from build123d import *

# Parameters (mm, degrees)
F1_DEPTH = 2
F2_SIZE  = 1


with BuildPart() as f1:
    # F0 (on Top) → F1 (new body, symmetric)
    with BuildSketch(Plane.XY):
        with BuildLine():
            Line((-64.3336782856, 36.2610286334), (-64.3336782856, 34.8834841531))
            Line((-64.3336782856, 34.8834841531), (-57.4157565349, 34.8834841531))
            Line((-57.4157565349, 34.8834841531), (-57.4157565349, 36.4834841531))
            ThreePointArc((-57.4157565349, 36.4834841531), (-56.2994751301, 38.665413461), (-55.5534152324, 41))
            Line((-55.5534152324, 41), (-53.1534152324, 41))
            Line((-53.1534152324, 41), (-53.1534152324, 42.5))
            Line((-53.1534152324, 42.5), (-43.6123318144, 42.5))
            Line((-43.6123318144, 42.5), (-43.6123318144, 45))
            Line((-43.6123318144, 45), (-43.6123318144, 47.5))
            Line((-43.6123318144, 47.5), (-53.1534152324, 47.5))
            Line((-53.1534152324, 47.5), (-53.1534152324, 49))
            Line((-53.1534152324, 49), (-55.5534152324, 49))
            ThreePointArc((-55.5534152324, 49), (-56.2994751301, 51.334586539), (-57.4157565349, 53.5165158469))
            Line((-57.4157565349, 53.5165158469), (-57.4157565349, 55.1165158469))
            Line((-57.4157565349, 55.1165158469), (-64.3336782856, 55.1165158469))
            Line((-64.3336782856, 55.1165158469), (-64.3336782856, 53.7389713666))
            ThreePointArc((-64.3336782856, 53.7389713666), (-61.2693193587, 50.1809672734), (-60.1668349206, 45.6165158469))
            Line((-60.1668349206, 45.6165158469), (-60.1668349206, 44.3834841531))
            ThreePointArc((-60.1668349206, 44.3834841531), (-61.2693193587, 39.8190327266), (-64.3336782856, 36.2610286334))
        make_face()
    extrude(amount=F1_DEPTH, both=True)

    # F2
    f2_edges = [f1.edges().sort_by_distance(p)[0] for p in [
        (-54.353415, 49, -2),
        (-54.353415, 49, 2),
        (-54.353415, 41, 2),
        (-54.353415, 41, -2),
        (-48.382874, 47.5, -2),
        (-48.382874, 42.5, -2),
        (-48.382874, 47.5, 2),
        (-48.382874, 42.5, 2),
        (-61.269319, 50.180967, 2),
        (-61.269319, 39.819033, -2),
        (-61.269319, 39.819033, 2),
        (-60.166835, 45, -2),
        (-60.166835, 45, 2),
        (-61.269319, 50.180967, -2),
    ]]
    chamfer(f2_edges, length=F2_SIZE)


solid = f1.part
Part model, mm, in its own coordinate system. A direction names the side the tool comes from. Coordinates: 2 decimals unless noted, no trailing zeros. Loops run counter-clockwise (first coordinate to the right, second up) from the corner with the lowest first, then second, coordinate; pieces in that order, holes last. Notation, with made-up numbers: (62, -31) -> (117, -31) arc R8 cw to (117, -19) -> close; hole circle Ø7 at (78, 44.25). An arc over 180 degrees is marked (long way). Use a Markdown table: item, result. Add a question column.
Item 1: Band-saw the part on A-A on x = -54.25. Write the cut outline in (y, z), plus the area to 3 significant figures.
Item 2: Which spindle directions (+Z, -Z, +X, -X, +Y, -Y) get a long thin tool onto all of the face, cutting with end or side? Do faces 5 (the flat face through (-48.4, 43, 1.5)), 6 (the flat face through (-54.3, 48.5, -1.5)), 7 (the flat face through (-48.4, 43, -1.5)), 8 (the flat face through (-54, 41, 0)), 9 (the flat face through (-60.167, 45, 0)). Say none if no direction does.
Item 3: Flat gauge pins, fed straight in: P1, Ø0.6, axis at x = -54.5, z = -0.5, coming from the +Y side; P2, Ø1, axis at x = -46.5, z = 0.5, coming from the +Y side; P3, Ø2, axis at y = 43, z = 0, coming from the -X side. Where does each tip first touch, or does it go through?
Item 4: Probe probe 1 along Y at (x, z) = (-55.5, 0.6); probe 2 along Y at (x, z) = (-45, 0); probe 3 along Y at (x, z) = (-62, 0.8). List the from-to ranges inside material, lowest first.
Item 5: Pull direction Y, two halves, no side cores. Call faces 1 (the flat face through (-54, 49, 0)), 2 (the flat face through (-57.416, 54, 0)), 3 (the cylindrical face through (-61.24, 39.88, 0.01)), 4 (the conical face through (-61.1, 39.5, 1.3)): +Y half, -Y half, draft (parallel to the pull), parting line (faces both ways), or undercut.
Item 6: Band-saw the part on C-C on z = 1.75. Write the cut outline in (x, y), plus the area to 3 significant figures.
Item 7: Band-saw the part on B-B on z = -0.05. Write the cut outline in (x, y).
Geometry says:
| question | item | result |
|---|---|---|
| 1 | outline | (41, -1) -> (42, -2) -> (48, -2) -> (49, -1) -> (49, 1) -> (48, 2) -> (42, 2) -> (41, 1) -> close |
| 1 | area | 30.0 mm² |
| 2 | face 5 | +Z, +X, -Y |
| 2 | face 6 | -Z, +X, +Y |
| 2 | face 7 | -Z, +X, -Y |
| 2 | face 8 | +Z, -Z, +X, -Y |
| 2 | face 9 | +Z, -Z, -X |
| 3 | P1 | y = 49 |
| 3 | P2 | y = 47.5 |
| 3 | P3 | x = -60.46 |
| 4 | probe 1 | 41 to 49 |
| 4 | probe 2 | 42.5 to 47.5 |
| 4 | probe 3 | 34.88 to 38.61, 51.39 to 55.12 |
| 5 | face 1 | +Y half |
| 5 | face 2 | draft |
| 5 | face 3 | undercut |
| 5 | face 4 | undercut |
| 6 | outline | (-64.33, 34.88) -> (-57.42, 34.88) -> (-57.42, 36.48) arc R15 ccw to (-55.4, 41.75) -> (-53.15, 41.75) -> (-53.15, 43.25) -> (-43.61, 43.25) -> (-43.61, 46.75) -> (-53.15, 46.75) -> (-53.15, 48.25) -> (-55.4, 48.25) arc R15 ccw to (-57.42, 53.52) -> (-57.42, 55.12) -> (-64.33, 55.12) -> (-64.33, 54.65) arc R10.75 cw to (-59.42, 45.62) -> (-59.42, 44.38) arc R10.75 cw to (-64.33, 35.35) -> close |
| 6 | area | 145 mm² |
| 7 | outline | (-64.33, 34.88) -> (-57.42, 34.88) -> (-57.42, 36.48) arc R15 ccw to (-55.55, 41) -> (-53.15, 41) -> (-53.15, 42.5) -> (-43.61, 42.5) -> (-43.61, 47.5) -> (-53.15, 47.5) -> (-53.15, 49) -> (-55.55, 49) arc R15 ccw to (-57.42, 53.52) -> (-57.42, 55.12) -> (-64.33, 55.12) -> (-64.33, 53.74) arc R10 cw to (-60.17, 45.62) -> (-60.17, 44.38) arc R10 cw to (-64.33, 36.26) -> close |
